Model file for the job. Use its own axes, mm. Coordinates: 2 decimals unless noted, no trailing zeros. Write each loop counter-clockwise with the first axis right and the second up, starting at its lowest first coordinate (ties: lowest second). Pieces come first, ordered by that corner, then holes. Notation, with made-up numbers: M 0,30.5 L 5,30.5 A21 ccw 5,63.5 Z; hole C 68.5,41 d10. An arc over 180 degrees is marked long. Put each result on its own line as item: value. Start each with the question number.
Q1. Drill centre lines: line 1 along Z through (x, y) = (0, 18.5); line 2 along Y through (x, z) = (8.25, 5); line 3 along X through (y, z) = (87, 0.5). Where is each one in solid material? Low to high.
Q2. Pull direction X, two halves, no side cores. Call faces 1 (the cylindrical face through (-1.08, 149.58, -4.88)), 2 (the flat face through (-2, 120, 5)), 3 (the flat face through (0, 30, 0)), 4 (the cylindrical face through (-3, 15, 0)): pulls with the +X half, pulls with the -X half, needs draft (parallel to the pull), parting line crosses it, or undercut.
Q3. Cut at A-A (z = 0). Write the cut outline in (x, y), then the cut area to 3 significant figures.
Q4. Drop flat-ended pins along their axis: pin 1 (4 mm diameter, centred on y = 60.5, z = -4, fed in from +X); pin 2 (6 mm diameter, centred on y = 48.5, z = -6.5, fed in from +X); pin 3 (2 mm diameter, centred on x = 2.5, y = 68, fed in from -Z). Give the stop position or say it passes through.
Q5. Cut at B-B (x = 0). Write the cut outline in (y, z).
Q6. Cut at C-C (z = 7.5). Write the cut outline in (x, y).
Autodesk Inventor part; units mm, degrees
ref_plane "YZ Plane" through (0, 0, 0) normal (1, 0, 0) x (0, 1, 0)
ref_plane "XZ Plane" through (0, 0, 0) normal (0, 1, 0) x (-1, 0, 0)
ref_plane "XY Plane" through (0, 0, 0) normal (0, 0, 1) x (1, 0, 0)
sketch "Sketch1" plane through (0, 0, 0) normal (0, 1, 0) x (-1, 0, 0)
  circle A0 centre (0, 0) radius 10
  dimension "d0" = 20
extrude "Extrusion1" add sketch "Sketch1" along normal blind 120
sketch "Sketch2" plane through (0, 120, 0) normal (0, 1, 0) x (1, 0, 0)
  circle A0 centre (0, 0) radius 5
  dimension "d3" = 10
extrude "Extrusion2" add sketch "Sketch2" along normal blind 60
thread "Thread1"
sketch "Sketch3" plane through (0, 0, 0) normal (0, -1, 0) x (1, 0, 0)
  circle A0 centre (0, 0) radius 3
  dimension "d8" = 6
extrude "Extrusion3" cut sketch "Sketch3" against normal blind 30
properties part number "center" material "Steel, Mild"
Computed values:
1. line 1: -10 to -3, 3 to 10
1. line 2: 0 to 120
1. line 3: -9.99 to 9.99
2. face 1: parting line crosses it
2. face 2: needs draft
2. face 3: undercut
2. face 4: undercut
3. outline: M -10,0 L -3,0 L -3,30 L 3,30 L 3,0 L 10,0 L 10,120 L 5,120 L 5,180 L -5,180 L -5,120 L -10,120 Z
3. area: 2,820 mm2
4. pin 1: x = 9.8
4. pin 2: x = 9.37
4. pin 3: z = -9.89
5. outline: M 0,-10 L 120,-10 L 120,-5 L 180,-5 L 180,5 L 120,5 L 120,10 L 0,10 L 0,3 L 30,3 L 30,-3 L 0,-3 Z
6. outline: M -6.61,0 L 6.61,0 L 6.61,120 L -6.61,120 Z
